The listing builds one solid part. Answer for the finished solid, in the listing's coordinates (mm). Round coordinates to 2 decimals unless told otherwise and drop trailing zeros. Write each loop counter-clockwise with the first axis right and the second up, starting at its lowest first coordinate (ties: lowest second). Pieces come first, ordered by that corner, then holes. Notation, with made-up numbers: M 15.25,72.5 L 73.25,72.5 A9 ccw 73.25,83.5 Z; hole C 68.25,26.5 d7. An arc over 180 degrees is marked long. One line per item, written item: value. Start each with the question number.
(1) Consider probe 1 along Z at (x, y) = (1.75, 7.5); probe 2 along Y at (x, z) = (2.4, -54.5); probe 3 along Z at (x, y) = (2.2, -100). Determine where each line is inside the solid, lowest interval first.
(2) Section A-A (z = -63.5) is taken. Determine the outline of the cut face in (x, y), plus the area to 3 significant figures.
(3) Given P1, Ø4, axis at y = 115.65, z = -100.8, coming from the +X side, flat-ended and moving along its own axis, determine where the tip first touches the part or whether it passes through.
Autodesk Inventor part; units mm, degrees
ref_plane "作業平面4" through (2.6, 125.6523, 179.1954) normal (0, -0.7071, 0.7071) x (-1, 0, 0)
ref_plane "作業平面5" through (0, -164.3477, 179.1954) normal (0, -0.7071, -0.7071) x (0, 0.7071, -0.7071)
ref_plane "YZ Plane" through (0, 0, 0) normal (1, 0, 0) x (0, 1, 0)
sketch "スケッチ1" plane through (0, 0, 0) normal (1, 0, 0) x (0, 1, 0)
  line L0 (125.6523, 179.1954) -> (-164.3477, 179.1954)
  line L1 (-164.3477, 179.1954) -> (-164.3477, -110.8046)
  line L2 (-164.3477, -110.8046) -> (125.6523, -110.8046)
  line L3 (125.6523, -110.8046) -> (125.6523, 179.1954)
  point P0 (0, 0)
  dimension "d0" = 290
  dimension "d1" = 290
extrude "押し出し1" add sketch "スケッチ1" along normal blind 2.6
sketch "スケッチ2" plane through (2.6, 0, 0) normal (1, 0, 0) x (0, 0, -1)
  line L0 (-179.1954, 125.6523) -> (-179.1954, -164.3477)
  line L1 (-179.1954, -164.3477) -> (110.8046, -164.3477)
  line L2 (110.8046, -164.3477) -> (110.8046, 125.6523)
  line L3 (110.8046, 125.6523) -> (-179.1954, 125.6523)
  line L4 (-34.1954, -19.3477) -> (-34.1954, 125.6523)
  line L5 (110.8046, 125.6523) -> (-179.1954, 125.6523)
  line L6 (-34.1954, -19.3477) -> (110.8046, -19.3477)
  point P0 (0, 0)
  point P1 (-169.1954, 115.6523)
  point P2 (100.8046, 115.6523)
  point P3 (-169.1954, -154.3477)
  point P4 (100.8046, -154.3477)
  dimension "d4" = 10
  dimension "d5" = 10
hole "穴1" at (2.6, 115.6523, 169.1954) at (2.6, 115.6523, -100.8046) at (2.6, -154.3477, 169.1954) at (2.6, -154.3477, -100.8046) direction (-1, 0, 0) diameter 4.5 depth 10 tip angle 118
sketch "スケッチ4" plane through (0, 0, 0) normal (-1, 0, 0) x (0, 0, 1)
  line L0 (179.1954, -164.3477) -> (-110.8046, -164.3477)
  line L1 (-110.8046, -164.3477) -> (-110.8046, 125.6523)
  line L2 (-110.8046, 126.1523) -> (179.1954, 126.1523)
  circle A0 centre (169.1954, -154.3477) radius 2.25
  circle A1 centre (169.1954, 115.6523) radius 2.25
  circle A2 centre (-100.8046, 115.6523) radius 2.25
  circle A3 centre (-100.8046, -154.3477) radius 2.25
  line L3 (179.1954, 125.6523) -> (179.1954, -164.3477)
  line L4 (-110.8046, 125.6523) -> (179.1954, 125.6523)
  line L5 (-110.8046, -164.3477) -> (-110.8046, 125.6523)
  line L6 (179.1954, -164.3477) -> (-110.8046, -164.3477)
  line L7 (179.1954, -164.3477) -> (-110.8046, -164.3477)
  line L8 (-70.8046, -152.3477) -> (-70.8046, -146.3477)
  line L9 (-68.8046, -144.3477) -> (-42.8046, -144.3477)
  line L10 (-40.8046, -146.3477) -> (-40.8046, -152.3477)
  arc A4 (-68.8046, -144.3477) -> (-70.8046, -146.3477) centre (-68.8046, -146.3477) ccw
  arc A5 (-40.8046, -146.3477) -> (-42.8046, -144.3477) centre (-42.8046, -146.3477) ccw
  line L11 (-42.8046, -154.3477) -> (-68.8046, -154.3477)
  arc A6 (-42.8046, -154.3477) -> (-40.8046, -152.3477) centre (-42.8046, -152.3477) ccw
  arc A7 (-70.8046, -152.3477) -> (-68.8046, -154.3477) centre (-68.8046, -152.3477) ccw
  arc A8 (109.1954, 107.6523) -> (111.1954, 105.6523) centre (111.1954, 107.6523) ccw
  line L12 (109.1954, 107.6523) -> (109.1954, 113.6523)
  arc A9 (111.1954, 115.6523) -> (109.1954, 113.6523) centre (111.1954, 113.6523) ccw
  line L13 (111.1954, 115.6523) -> (137.1954, 115.6523)
  line L14 (137.1954, 105.6523) -> (111.1954, 105.6523)
  arc A10 (137.1954, 105.6523) -> (139.1954, 107.6523) centre (137.1954, 107.6523) ccw
  line L15 (139.1954, 113.6523) -> (139.1954, 107.6523)
  arc A11 (139.1954, 113.6523) -> (137.1954, 115.6523) centre (137.1954, 113.6523) ccw
  point P0 (0, 0)
  point P1 (-70.8046, -164.3477)
  point P2 (-70.8046, -144.3477)
  point P3 (-40.8046, -144.3477)
  point P4 (-40.8046, -164.3477)
  point P5 (34.1954, -19.3477)
  point P6 (109.1954, 105.6523)
  point P7 (109.1954, 125.6523)
  point P8 (139.1954, 105.6523)
  point P9 (139.1954, 125.6523)
  dimension "d19" = 40
  dimension "d20" = 30
  dimension "d21" = 20
  dimension "d22" = 2
  dimension "d23" = 10
  dimension "d24" = 2
  dimension "d25" = 145
  dimension "d26" = 145
  dimension "d29" = 360
extrude "押し出し3" cut sketch "スケッチ4" against normal blind 2.6 contours L8 A4 L9 A5 L10 A6 L11 A7 | L12 A9 L13 A11 L15 A10 L14 A8
ref_plane "作業平面4" through (2.6, 125.6523, 179.1954) normal (0, -0.7071, 0.7071) x (-1, 0, 0)
ref_plane "作業平面5" through (0, -164.3477, 179.1954) normal (0, -0.7071, -0.7071) x (0, 0.7071, -0.7071)
sketch "スケッチ5" plane through (0, 0, 0) normal (-1, 0, 0) x (0, 0, 1)
  circle A0 centre (60.7119, 60.2018) radius 1.65
  circle A1 centre (113.7449, 7.1688) radius 1.65
  circle A2 centre (-45.3541, -45.8642) radius 1.65
  circle A3 centre (7.6789, -98.8972) radius 1.65
  circle A4 centre (7.6789, -98.8972) radius 1.65
  circle A5 centre (7.6789, -98.8972) radius 1.65
  point P0 (0, 0)
hole "穴2" at (0, 7.1688, 113.7449) at (0, -98.8972, 7.6789) at (0, -45.8642, -45.3541) at (0, 60.2018, 60.7119) at (0, 7.1688, 113.7449) direction (1, 0, 0) diameter 4.5 end through all
properties part number "lc_box_side" material "ポリカーボネート、クリア"
Recorded:
1. probe 1: z = -110.8 to 111.52, 115.97 to 179.2
1. probe 2: y = -164.35 to -154.35, -144.35 to 125.65
1. probe 3: z = -110.8 to 5.72, 9.64 to 179.2
2. outline: M 0,-164.35 L 2.6,-164.35 L 2.6,-154.35 L 0,-154.35 Z; M 0,-144.35 L 2.6,-144.35 L 2.6,125.65 L 0,125.65 Z
2. area: 728 mm2
3. P1: passes through
